The listing builds one solid part. Answer for the finished solid, in the listing's coordinates (mm). A direction names the side the tool comes from. Give positions to 0.01 mm unless a question says otherwise; leave off trailing zeros. Loops run counter-clockwise (first coordinate to the right, second up) from the corner with the lowest first, then second, coordinate; pieces in that order, holes last.
Item 1: Section B-B, the plane y = 4.5 is taken. Give the number of separate pieces and of enclosed holes in the cut face, and give its area (3 significant figures).
Item 2: Section C-C, the plane z = -25.5 is taken. Give the vertices of the cut face in (x, y).
Item 3: The mould has two halves that part along Z. Classify faces 1 (the face through (-3, 9, 45)), 2 (the face through (-7.07, -1.52, -2.02)), 3 (the face through (44.717, 5.198, 38.647)): pulls with the +Z half, pulls with the -Z half, needs draft (parallel to the pull), parting line crosses it, or undercut.
Item 4: Section A-A, the plane x = 22.5 is taken. Give the vertices of the cut face in (y, z).
Item 5: A tool of negligible diameter and unlimited length cuts with its end or side. For faces 4 (the face through (43, 5, -1)), 5 (the face through (38, 1.5, -47)), 6 (the face through (39, 5, -44.8)), 7 (the face through (36, -1, 29.24)), 8 (the face through (40.8, 5, 39)), from which of +Z, -Z, +X, -X, +Y, -Y can it reach the whole face along a straight path? Write none if from no direction.
Item 6: Each of these flat-tipped pins is pushed along its axis until it touches: pin 1 Ø2.5 at (x, y) = (39, 6.5) entering from +Z; pin 2 Ø0.9 at (x, y) = (-40.5, -1.5) entering from -Z; pin 3 Ø0.8 at (x, y) = (-45, 4.5) entering from +Z; pin 4 Ø3 at (x, z) = (-12.5, 3) entering from -Y. Where does it stop, or does it pass through?
Item 7: Consider line 1 along Z through (x, y) = (12, 1.5); line 2 along X through (y, z) = (-2.25, -27); line 3 along Z through (x, y) = (-19.5, -1.75). Determine where each line is inside the solid, lowest interval first.
from build123d import *

# Parameters (mm, degrees)
BASE_FLANGE1_DEPTH             = 3
FILLET1_R                      = 2
EDGE_FLANGE1_STRIP_W           = 15
EDGE_FLANGE1_STRIP_H           = 3
EDGE_FLANGE1_STRIP_CUT_DEPTH   = 74.48
EDGE_FLANGE1_STRIP_2_W         = 15
EDGE_FLANGE1_STRIP_2_H         = 3
EDGE_FLANGE1_STRIP_CUT_2_DEPTH = 74.48
EDGE_FLANGE1_STRIP_3_W         = 15
EDGE_FLANGE1_STRIP_3_H         = 3
EDGE_FLANGE1_STRIP_CUT_3_DEPTH = 74.48
EDGE_FLANGE1_STRIP_4_W         = 15
EDGE_FLANGE1_STRIP_4_H         = 3
EDGE_FLANGE1_STRIP_CUT_4_DEPTH = 74.48
EDGE_FLANGE1_DEPTH             = 74.48
EDGE_FLANGE1_BEND_DEPTH        = 74.48
EDGE_FLANGE1_BEND_2_DEPTH      = 74.48
EDGE_FLANGE1_BEND_3_DEPTH      = 74.48
EDGE_FLANGE2_DEPTH             = 7.5
EDGE_FLANGE2_BEND_DEPTH        = 7.5
EDGE_FLANGE2_BEND_2_DEPTH      = 7.5
EDGE_FLANGE2_BEND_3_DEPTH      = 7.5
EDGE_FLANGE2_BEND_4_DEPTH      = 7.5
EDGE_FLANGE2_BEND_5_DEPTH      = 7.5
EDGE_FLANGE2_BEND_6_DEPTH      = 7.5
EDGE_FLANGE2_BEND_7_DEPTH      = 7.5


# Sheet-metal steps are written as plain solids
with BuildPart() as part:
    # Sketch1 → Base-Flange1 (new body)
    with BuildSketch(Plane(origin=(0, 0, 0), x_dir=(1, 0, 0), z_dir=(0, 1, 0))):
        Polygon((-50, 39.24), (-39.24, 39.24), (-39.24, 50), (35.24, 50), (35.24, 39.24), (46, 39.24), (46, -35.24), (35.24, -35.24), (35.24, -46), (-39.24, -46), (-39.24, -35.24), (-50, -35.24), align=None)
        Polygon((-37.482640687, 33.24), (-6.242640687, 2), (-37.482640687, -29.24), (-44, -29.24), (-44, 33.24), align=None, mode=Mode.SUBTRACT)
        Polygon((-33.24, 37.482640687), (-2, 6.242640687), (29.24, 37.482640687), (29.24, 44), (-33.24, 44), align=None, mode=Mode.SUBTRACT)
        Polygon((33.482640687, 33.24), (2.242640687, 2), (33.482640687, -29.24), (40, -29.24), (40, 33.24), align=None, mode=Mode.SUBTRACT)
        Polygon((-33.24, -40), (-33.24, -33.482640687), (-2, -2.242640687), (29.24, -33.482640687), (29.24, -40), align=None, mode=Mode.SUBTRACT)
    extrude(amount=-BASE_FLANGE1_DEPTH)

    # Fillet1
    fillet1_edges = [part.edges().sort_by_distance(p)[0] for p in [
        (29.24, -1.5, -44),
        (29.24, -1.5, -37.482640687),
        (-2, -1.5, -6.242640687),
        (-33.24, -1.5, -37.482640687),
        (-33.24, -1.5, -44),
        (-44, -1.5, 29.24),
        (-44, -1.5, -33.24),
        (-37.482640687, -1.5, -33.24),
        (-6.242640687, -1.5, -2),
        (-37.482640687, -1.5, 29.24),
        (29.24, -1.5, 40),
        (-33.24, -1.5, 40),
        (-33.24, -1.5, 33.482640687),
        (-2, -1.5, 2.242640687),
        (29.24, -1.5, 33.482640687),
        (40, -1.5, -33.24),
        (40, -1.5, 29.24),
        (33.482640687, -1.5, 29.24),
        (2.242640687, -1.5, -2),
        (33.482640687, -1.5, -33.24),
    ]]
    fillet(fillet1_edges, radius=FILLET1_R)

    # Edge-Flange1 strip (across the edge) → Edge-Flange1 strip cut (cut)
    with BuildSketch(Plane(origin=(-50, 0, -39.24), x_dir=(1, 0, 0), z_dir=(0, 0, 1))):
        with Locations((-3, -1.5)):
            Rectangle(EDGE_FLANGE1_STRIP_W, EDGE_FLANGE1_STRIP_H)
    extrude(amount=EDGE_FLANGE1_STRIP_CUT_DEPTH, mode=Mode.SUBTRACT)

    # Edge-Flange1 strip 2 (across the edge) → Edge-Flange1 strip cut 2 (cut)
    with BuildSketch(Plane(origin=(46, 0, 35.24), x_dir=(-1, 0, 0), z_dir=(0, 0, -1))):
        with Locations((-3, -1.5)):
            Rectangle(EDGE_FLANGE1_STRIP_2_W, EDGE_FLANGE1_STRIP_2_H)
    extrude(amount=EDGE_FLANGE1_STRIP_CUT_2_DEPTH, mode=Mode.SUBTRACT)

    # Edge-Flange1 strip 3 (across the edge) → Edge-Flange1 strip cut 3 (cut)
    with BuildSketch(Plane(origin=(-39.24, 0, 46), x_dir=(0, 0, -1), z_dir=(1, 0, 0))):
        with Locations((-3, -1.5)):
            Rectangle(EDGE_FLANGE1_STRIP_3_W, EDGE_FLANGE1_STRIP_3_H)
    extrude(amount=EDGE_FLANGE1_STRIP_CUT_3_DEPTH, mode=Mode.SUBTRACT)

    # Edge-Flange1 strip 4 (across the edge) → Edge-Flange1 strip cut 4 (cut)
    with BuildSketch(Plane(origin=(35.24, 0, -50), x_dir=(0, 0, 1), z_dir=(-1, 0, 0))):
        with Locations((-3, -1.5)):
            Rectangle(EDGE_FLANGE1_STRIP_4_W, EDGE_FLANGE1_STRIP_4_H)
    extrude(amount=EDGE_FLANGE1_STRIP_CUT_4_DEPTH, mode=Mode.SUBTRACT)

    # Edge-Flange1 section (across the edge) → Edge-Flange1 (add)
    with BuildSketch(Plane(origin=(-50, 0, -39.24), x_dir=(1, 0, 0), z_dir=(0, 0, 1))):
        with BuildLine():
            Line((0, 1.5), (0, 9))
            Line((0, 9), (3, 9))
            Line((3, 9), (3, 1.5))
            ThreePointArc((3, 1.5), (3.439339828, 0.439339828), (4.5, 0))
            Line((4.5, 0), (4.5, -3))
            ThreePointArc((4.5, -3), (1.318019485, -1.681980515), (0, 1.5))
        make_face()
    extrude(amount=EDGE_FLANGE1_DEPTH)

    # Edge-Flange1 section 2 (across the edge) → Edge-Flange1 bend (add)
    with BuildSketch(Plane(origin=(46, 0, 35.24), x_dir=(-1, 0, 0), z_dir=(0, 0, -1))):
        with BuildLine():
            Line((0, 1.5), (0, 9))
            Line((0, 9), (3, 9))
            Line((3, 9), (3, 1.5))
            ThreePointArc((3, 1.5), (3.439339828, 0.439339828), (4.5, 0))
            Line((4.5, 0), (4.5, -3))
            ThreePointArc((4.5, -3), (1.318019485, -1.681980515), (0, 1.5))
        make_face()
    extrude(amount=EDGE_FLANGE1_BEND_DEPTH)

    # Edge-Flange1 section 3 (across the edge) → Edge-Flange1 bend 2 (add)
    with BuildSketch(Plane(origin=(-39.24, 0, 46), x_dir=(0, 0, -1), z_dir=(1, 0, 0))):
        with BuildLine():
            Line((0, 1.5), (0, 9))
            Line((0, 9), (3, 9))
            Line((3, 9), (3, 1.5))
            ThreePointArc((3, 1.5), (3.439339828, 0.439339828), (4.5, 0))
            Line((4.5, 0), (4.5, -3))
            ThreePointArc((4.5, -3), (1.318019485, -1.681980515), (0, 1.5))
        make_face()
    extrude(amount=EDGE_FLANGE1_BEND_2_DEPTH)

    # Edge-Flange1 section 4 (across the edge) → Edge-Flange1 bend 3 (add)
    with BuildSketch(Plane(origin=(35.24, 0, -50), x_dir=(0, 0, 1), z_dir=(-1, 0, 0))):
        with BuildLine():
            Line((0, 1.5), (0, 9))
            Line((0, 9), (3, 9))
            Line((3, 9), (3, 1.5))
            ThreePointArc((3, 1.5), (3.439339828, 0.439339828), (4.5, 0))
            Line((4.5, 0), (4.5, -3))
            ThreePointArc((4.5, -3), (1.318019485, -1.681980515), (0, 1.5))
        make_face()
    extrude(amount=EDGE_FLANGE1_BEND_3_DEPTH)

    # Edge-Flange2 section (across the edge) → Edge-Flange2 (add)
    with BuildSketch(Plane(origin=(43, 9, -41), x_dir=(0, 0, 1), z_dir=(0, -1, 0))):
        with BuildLine():
            Line((-3, 1.5), (-3, 2.2))
            Line((-3, 2.2), (0, 2.2))
            Line((0, 2.2), (0, 1.5))
            ThreePointArc((0, 1.5), (0.439339828, 0.439339828), (1.5, 0))
            Line((1.5, 0), (1.76, 0))
            Line((1.76, 0), (1.76, -3))
            Line((1.76, -3), (1.5, -3))
            ThreePointArc((1.5, -3), (-1.681980515, -1.681980515), (-3, 1.5))
        make_face()
    extrude(amount=EDGE_FLANGE2_DEPTH)

    # Edge-Flange2 section 2 (across the edge) → Edge-Flange2 bend (add)
    with BuildSketch(Plane(origin=(37, 1.5, -47), x_dir=(-1, 0, 0), z_dir=(0, 1, 0))):
        with BuildLine():
            Line((-3, 1.5), (-3, 2.2))
            Line((-3, 2.2), (0, 2.2))
            Line((0, 2.2), (0, 1.5))
            ThreePointArc((0, 1.5), (0.439339828, 0.439339828), (1.5, 0))
            Line((1.5, 0), (1.76, 0))
            Line((1.76, 0), (1.76, -3))
            Line((1.76, -3), (1.5, -3))
            ThreePointArc((1.5, -3), (-1.681980515, -1.681980515), (-3, 1.5))
        make_face()
    extrude(amount=EDGE_FLANGE2_BEND_DEPTH)

    # Edge-Flange2 section 3 (across the edge) → Edge-Flange2 bend 2 (add)
    with BuildSketch(Plane(origin=(-41, 9, -47), x_dir=(1, 0, 0), z_dir=(0, -1, 0))):
        with BuildLine():
            Line((-3, 1.5), (-3, 2.2))
            Line((-3, 2.2), (0, 2.2))
            Line((0, 2.2), (0, 1.5))
            ThreePointArc((0, 1.5), (0.439339828, 0.439339828), (1.5, 0))
            Line((1.5, 0), (1.76, 0))
            Line((1.76, 0), (1.76, -3))
            Line((1.76, -3), (1.5, -3))
            ThreePointArc((1.5, -3), (-1.681980515, -1.681980515), (-3, 1.5))
        make_face()
    extrude(amount=EDGE_FLANGE2_BEND_2_DEPTH)

    # Edge-Flange2 section 4 (across the edge) → Edge-Flange2 bend 3 (add)
    with BuildSketch(Plane(origin=(-47, 1.5, -41), x_dir=(0, 0, 1), z_dir=(0, 1, 0))):
        with BuildLine():
            Line((-3, 1.5), (-3, 2.2))
            Line((-3, 2.2), (0, 2.2))
            Line((0, 2.2), (0, 1.5))
            ThreePointArc((0, 1.5), (0.439339828, 0.439339828), (1.5, 0))
            Line((1.5, 0), (1.76, 0))
            Line((1.76, 0), (1.76, -3))
            Line((1.76, -3), (1.5, -3))
            ThreePointArc((1.5, -3), (-1.681980515, -1.681980515), (-3, 1.5))
        make_face()
    extrude(amount=EDGE_FLANGE2_BEND_3_DEPTH)

    # Edge-Flange2 section 5 (across the edge) → Edge-Flange2 bend 4 (add)
    with BuildSketch(Plane(origin=(-47, 9, 37), x_dir=(0, 0, -1), z_dir=(0, -1, 0))):
        with BuildLine():
            Line((-3, 1.5), (-3, 2.2))
            Line((-3, 2.2), (0, 2.2))
            Line((0, 2.2), (0, 1.5))
            ThreePointArc((0, 1.5), (0.439339828, 0.439339828), (1.5, 0))
            Line((1.5, 0), (1.76, 0))
            Line((1.76, 0), (1.76, -3))
            Line((1.76, -3), (1.5, -3))
            ThreePointArc((1.5, -3), (-1.681980515, -1.681980515), (-3, 1.5))
        make_face()
    extrude(amount=EDGE_FLANGE2_BEND_4_DEPTH)

    # Edge-Flange2 section 6 (across the edge) → Edge-Flange2 bend 5 (add)
    with BuildSketch(Plane(origin=(-41, 1.5, 43), x_dir=(1, 0, 0), z_dir=(0, 1, 0))):
        with BuildLine():
            Line((-3, 1.5), (-3, 2.2))
            Line((-3, 2.2), (0, 2.2))
            Line((0, 2.2), (0, 1.5))
            ThreePointArc((0, 1.5), (0.439339828, 0.439339828), (1.5, 0))
            Line((1.5, 0), (1.76, 0))
            Line((1.76, 0), (1.76, -3))
            Line((1.76, -3), (1.5, -3))
            ThreePointArc((1.5, -3), (-1.681980515, -1.681980515), (-3, 1.5))
        make_face()
    extrude(amount=EDGE_FLANGE2_BEND_5_DEPTH)

    # Edge-Flange2 section 7 (across the edge) → Edge-Flange2 bend 6 (add)
    with BuildSketch(Plane(origin=(37, 9, 43), x_dir=(-1, 0, 0), z_dir=(0, -1, 0))):
        with BuildLine():
            Line((-3, 1.5), (-3, 2.2))
            Line((-3, 2.2), (0, 2.2))
            Line((0, 2.2), (0, 1.5))
            ThreePointArc((0, 1.5), (0.439339828, 0.439339828), (1.5, 0))
            Line((1.5, 0), (1.76, 0))
            Line((1.76, 0), (1.76, -3))
            Line((1.76, -3), (1.5, -3))
            ThreePointArc((1.5, -3), (-1.681980515, -1.681980515), (-3, 1.5))
        make_face()
    extrude(amount=EDGE_FLANGE2_BEND_6_DEPTH)

    # Edge-Flange2 section 8 (across the edge) → Edge-Flange2 bend 7 (add)
    with BuildSketch(Plane(origin=(43, 1.5, 37), x_dir=(0, 0, -1), z_dir=(0, 1, 0))):
        with BuildLine():
            Line((-3, 1.5), (-3, 2.2))
            Line((-3, 2.2), (0, 2.2))
            Line((0, 2.2), (0, 1.5))
            ThreePointArc((0, 1.5), (0.439339828, 0.439339828), (1.5, 0))
            Line((1.5, 0), (1.76, 0))
            Line((1.76, 0), (1.76, -3))
            Line((1.76, -3), (1.5, -3))
            ThreePointArc((1.5, -3), (-1.681980515, -1.681980515), (-3, 1.5))
        make_face()
    extrude(amount=EDGE_FLANGE2_BEND_7_DEPTH)


solid = part.part
Worked answers:
1. separate pieces: 4
1. enclosed holes: 0
1. area: 1,030 mm2
2. outline: (-50, 1.5) arc R4.5 ccw to (-45.5, -3) - (-44, -3) - (-44, 0) - (-45.5, 0) arc R1.5 cw to (-47, 1.5) - (-47, 9) - (-50, 9) - close; (-29.74, -3) - (-21.26, -3) - (-21.26, 0) - (-29.74, 0) - close; (17.26, -3) - (25.74, -3) - (25.74, 0) - (17.26, 0) - close; (40, -3) - (41.5, -3) arc R4.5 ccw to (46, 1.5) - (46, 9) - (43, 9) - (43, 1.5) arc R1.5 cw to (41.5, 0) - (40, 0) - close
3. face 1: needs draft
3. face 2: undercut
3. face 3: pulls with the +Z half
4. outline: (-3, -45.5) arc R4.5 ccw to (1.5, -50) - (9, -50) - (9, -47) - (1.5, -47) arc R1.5 cw to (0, -45.5) - (0, -44) - (-3, -44) - close; (-3, -30.74) - (0, -30.74) - (0, -22.26) - (-3, -22.26) - close; (-3, 18.26) - (0, 18.26) - (0, 26.74) - (-3, 26.74) - close; (-3, 40) - (0, 40) - (0, 41.5) arc R1.5 cw to (1.5, 43) - (9, 43) - (9, 46) - (1.5, 46) arc R4.5 ccw to (-3, 41.5) - close
5. face 4: +Y
5. face 5: +Z, -Z, +X, -Y
5. face 6: +X, -X, +Y, -Y
5. face 7: +Y, -Y
5. face 8: +Z, -Z, +Y, -Y
6. pin 1: stops at z = 45.4
6. pin 2: stops at z = -39.24
6. pin 3: stops at z = 40
6. pin 4: stops at y = -3
7. line 1: z = -50 to -47, 43 to 46
7. line 2: x = -47.99 to -44, -31.24 to -22.76, 18.76 to 27.24, 40 to 43.99
7. line 3: z = -48.61 to -44, -23.74 to -15.26, 11.26 to 19.74, 40 to 44.61
